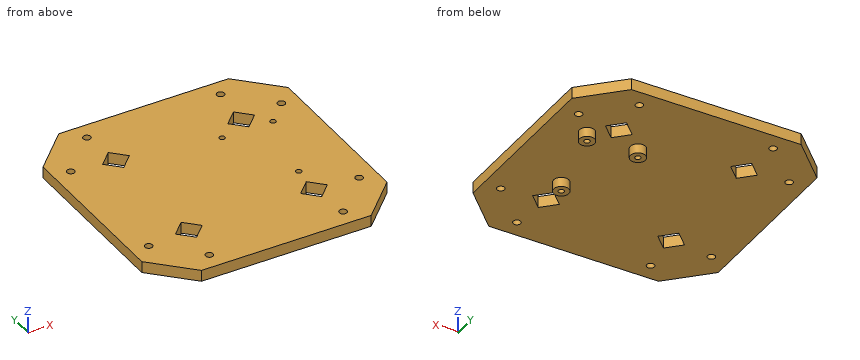
```python
from build123d import *

# Parameters (mm, degrees)
SKETCH_1_W          = 130
SKETCH_1_H          = 130
EXTRUDE_1_DEPTH     = 6
CUT_EXTRUDE_1_DEPTH = 6
CUT_EXTRUDE_2_REACH = 185.946
SKETCH_11_R         = 2
CHAMFER_1_SIZE      = 20
CUT_EXTRUDE_3_REACH = 185.946
SKETCH_12_R         = 1.5
SKETCH_13_R         = 4
SKETCH_13_R_2       = 1.5
EXTRUDE_2_DEPTH     = 5


with BuildPart() as part:
    # 草圖1 → 填料-伸長1 (new body)
    with BuildSketch(Plane.XY):
        with Locations((-65, 65)):
            Rectangle(SKETCH_1_W, SKETCH_1_H)
    extrude(amount=EXTRUDE_1_DEPTH)

    # 草圖10 → 除料-伸長1 (cut)
    with BuildSketch(Plane.XY.offset(6)):
        Polygon((-38.890872965, 98.180194847), (-31.819805153, 105.251262658), (-24.748737342, 98.180194847), (-31.819805153, 91.109127035), align=None)
        Polygon((-98.180194847, 105.251262658), (-105.251262658, 98.180194847), (-98.180194847, 91.109127035), (-91.109127035, 98.180194847), align=None)
        Polygon((-91.109127035, 31.819805153), (-98.180194847, 24.748737342), (-105.251262658, 31.819805153), (-98.180194847, 38.890872965), align=None)
        Polygon((-31.819805153, 24.748737342), (-24.748737342, 31.819805153), (-31.819805153, 38.890872965), (-38.890872965, 31.819805153), align=None)
    extrude(amount=-CUT_EXTRUDE_1_DEPTH, mode=Mode.SUBTRACT)

    # 草圖11 → 除料-伸長2 (cut, up to next)
    with BuildSketch(Plane.XY.offset(6), mode=Mode.PRIVATE) as cut_extrude_2_sk1:
        with Locations((-9.2, 100.435324702)):
            Circle(SKETCH_11_R)
    cut_extrude_2_tool1 = extrude(cut_extrude_2_sk1.sketch, amount=-CUT_EXTRUDE_2_REACH, mode=Mode.PRIVATE) & part.part
    # 草圖11 → 除料-伸長2 (cut, up to next)
    with BuildSketch(Plane.XY.offset(6), mode=Mode.PRIVATE) as cut_extrude_2_sk2:
        with Locations((-29.564675298, 120.8)):
            Circle(SKETCH_11_R)
    cut_extrude_2_tool2 = extrude(cut_extrude_2_sk2.sketch, amount=-CUT_EXTRUDE_2_REACH, mode=Mode.PRIVATE) & part.part
    # 草圖11 → 除料-伸長2 (cut, up to next)
    with BuildSketch(Plane.XY.offset(6), mode=Mode.PRIVATE) as cut_extrude_2_sk3:
        with Locations((-100.435324702, 120.8)):
            Circle(SKETCH_11_R)
    cut_extrude_2_tool3 = extrude(cut_extrude_2_sk3.sketch, amount=-CUT_EXTRUDE_2_REACH, mode=Mode.PRIVATE) & part.part
    # 草圖11 → 除料-伸長2 (cut, up to next)
    with BuildSketch(Plane.XY.offset(6), mode=Mode.PRIVATE) as cut_extrude_2_sk4:
        with Locations((-120.8, 100.435324702)):
            Circle(SKETCH_11_R)
    cut_extrude_2_tool4 = extrude(cut_extrude_2_sk4.sketch, amount=-CUT_EXTRUDE_2_REACH, mode=Mode.PRIVATE) & part.part
    # 草圖11 → 除料-伸長2 (cut, up to next)
    with BuildSketch(Plane.XY.offset(6), mode=Mode.PRIVATE) as cut_extrude_2_sk5:
        with Locations((-120.8, 29.564675298)):
            Circle(SKETCH_11_R)
    cut_extrude_2_tool5 = extrude(cut_extrude_2_sk5.sketch, amount=-CUT_EXTRUDE_2_REACH, mode=Mode.PRIVATE) & part.part
    # 草圖11 → 除料-伸長2 (cut, up to next)
    with BuildSketch(Plane.XY.offset(6), mode=Mode.PRIVATE) as cut_extrude_2_sk6:
        with Locations((-100.435324702, 9.2)):
            Circle(SKETCH_11_R)
    cut_extrude_2_tool6 = extrude(cut_extrude_2_sk6.sketch, amount=-CUT_EXTRUDE_2_REACH, mode=Mode.PRIVATE) & part.part
    # 草圖11 → 除料-伸長2 (cut, up to next)
    with BuildSketch(Plane.XY.offset(6), mode=Mode.PRIVATE) as cut_extrude_2_sk7:
        with Locations((-29.564675298, 9.2)):
            Circle(SKETCH_11_R)
    cut_extrude_2_tool7 = extrude(cut_extrude_2_sk7.sketch, amount=-CUT_EXTRUDE_2_REACH, mode=Mode.PRIVATE) & part.part
    # 草圖11 → 除料-伸長2 (cut, up to next)
    with BuildSketch(Plane.XY.offset(6), mode=Mode.PRIVATE) as cut_extrude_2_sk8:
        with Locations((-9.2, 29.564675298)):
            Circle(SKETCH_11_R)
    cut_extrude_2_tool8 = extrude(cut_extrude_2_sk8.sketch, amount=-CUT_EXTRUDE_2_REACH, mode=Mode.PRIVATE) & part.part
    add(cut_extrude_2_tool1.solids().sort_by_distance((-9.2, 100.435325, 6))[0], mode=Mode.SUBTRACT)
    add(cut_extrude_2_tool2.solids().sort_by_distance((-29.564675, 120.8, 6))[0], mode=Mode.SUBTRACT)
    add(cut_extrude_2_tool3.solids().sort_by_distance((-100.435325, 120.8, 6))[0], mode=Mode.SUBTRACT)
    add(cut_extrude_2_tool4.solids().sort_by_distance((-120.8, 100.435325, 6))[0], mode=Mode.SUBTRACT)
    add(cut_extrude_2_tool5.solids().sort_by_distance((-120.8, 29.564675, 6))[0], mode=Mode.SUBTRACT)
    add(cut_extrude_2_tool6.solids().sort_by_distance((-100.435325, 9.2, 6))[0], mode=Mode.SUBTRACT)
    add(cut_extrude_2_tool7.solids().sort_by_distance((-29.564675, 9.2, 6))[0], mode=Mode.SUBTRACT)
    add(cut_extrude_2_tool8.solids().sort_by_distance((-9.2, 29.564675, 6))[0], mode=Mode.SUBTRACT)

    # 導角1
    chamfer_1_edges = [part.edges().sort_by_distance(p)[0] for p in [
        (-130, 0, 3),
        (-130, 130, 3),
        (0, 130, 3),
        (0, 0, 3),
    ]]
    chamfer(chamfer_1_edges, length=CHAMFER_1_SIZE)

    # 草圖12 → 除料-伸長3 (cut, up to next)
    with BuildSketch(Plane.XY.offset(6), mode=Mode.PRIVATE) as cut_extrude_3_sk1:
        with Locations((-47, 89.5)):
            Circle(SKETCH_12_R)
    cut_extrude_3_tool1 = extrude(cut_extrude_3_sk1.sketch, amount=-CUT_EXTRUDE_3_REACH, mode=Mode.PRIVATE) & part.part
    # 草圖12 → 除料-伸長3 (cut, up to next)
    with BuildSketch(Plane.XY.offset(6), mode=Mode.PRIVATE) as cut_extrude_3_sk2:
        with Locations((-20, 89.5)):
            Circle(SKETCH_12_R)
    cut_extrude_3_tool2 = extrude(cut_extrude_3_sk2.sketch, amount=-CUT_EXTRUDE_3_REACH, mode=Mode.PRIVATE) & part.part
    # 草圖12 → 除料-伸長3 (cut, up to next)
    with BuildSketch(Plane.XY.offset(6), mode=Mode.PRIVATE) as cut_extrude_3_sk3:
        with Locations((-30.5, 48)):
            Circle(SKETCH_12_R)
    cut_extrude_3_tool3 = extrude(cut_extrude_3_sk3.sketch, amount=-CUT_EXTRUDE_3_REACH, mode=Mode.PRIVATE) & part.part
    add(cut_extrude_3_tool1.solids().sort_by_distance((-47, 89.5, 6))[0], mode=Mode.SUBTRACT)
    add(cut_extrude_3_tool2.solids().sort_by_distance((-20, 89.5, 6))[0], mode=Mode.SUBTRACT)
    add(cut_extrude_3_tool3.solids().sort_by_distance((-30.5, 48, 6))[0], mode=Mode.SUBTRACT)

    # 草圖13 → 填料-伸長2 (add)
    # profile 1 of 3: a face of its own
    with BuildSketch(Plane(origin=(0, 0, 0), x_dir=(-1, 0, 0), z_dir=(0, 0, -1))):
        with Locations(Location((20, 89.5, 0), (0, 0, 180))):
            Circle(SKETCH_13_R)
        with Locations(Location((20, 89.5, 0), (0, 0, 180))):
            Circle(SKETCH_13_R_2, mode=Mode.SUBTRACT)
    # profile 2 of 3: a face of its own
    with BuildSketch(Plane(origin=(0, 0, 0), x_dir=(-1, 0, 0), z_dir=(0, 0, -1))):
        with Locations(Location((47, 89.5, 0), (0, 0, 180))):
            Circle(SKETCH_13_R)
        with Locations(Location((47, 89.5, 0), (0, 0, 180))):
            Circle(SKETCH_13_R_2, mode=Mode.SUBTRACT)
    # profile 3 of 3: a face of its own
    with BuildSketch(Plane(origin=(0, 0, 0), x_dir=(-1, 0, 0), z_dir=(0, 0, -1))):
        with Locations(Location((30.5, 48, 0), (0, 0, 180))):
            Circle(SKETCH_13_R)
        with Locations(Location((30.5, 48, 0), (0, 0, 180))):
            Circle(SKETCH_13_R_2, mode=Mode.SUBTRACT)
    extrude(amount=EXTRUDE_2_DEPTH)


solid = part.part
```
The model under review builds one solid part; all positions refer to its coordinate system, in mm. Round coordinates to 2 decimals unless told otherwise and drop trailing zeros. Write each loop counter-clockwise with the first axis right and the second up, starting at its lowest first coordinate (ties: lowest second). Pieces come first, ordered by that corner, then holes. Notation, with made-up numbers: M 9,74 L 29,74 A28 cw 29,111 Z; hole C 58,-14.75 d1. An arc over 180 degrees is marked long. Use CSV: the item, a comma, the result in double quotes. Start each with the question number.
(1) We need section D-D, the plane x = -47. State the section outline as (y, z) points, then the cut area to 3 significant figures.
(2) Clearance check with flat-ended pins moving along their axes: P1, Ø4.5, axis at x = -29.56, y = 9.2, coming from the +Z side; P2, Ø5, axis at x = -17, z = 2, coming from the -Y side; P3, Ø5, axis at x = -29.56, y = 120.8, coming from the -Z side. State where each tip first meets the part, or that it passes through.
(3) We need section B-B, the plane y = 89.5. State the section outline as (x, z) points.
(4) We need section A-A, the plane x = -9.2. State the section outline as (y, z) points, then the cut area to 3 significant figures.
(5) We need section C-C, the plane z = -3. State the section outline as (x, y) points.
(6) For line 1 along X through (y, z) = (48, -2.65); line 2 along X through (y, z) = (120.5, 4.25); line 3 along Y through (x, z) = (-35.5, 1.25), list the stretches that pass through material, from the lowest coordinate up.
Findings:
1,outline,"M 0,0 L 85.5,0 L 85.5,-5 L 88,-5 L 88,6 L 0,6 Z; M 91,-5 L 93.5,-5 L 93.5,0 L 130,0 L 130,6 L 91,6 Z"
1,area,"787 mm^2"
2,P1,"z = 6"
2,P2,"y = 0.5"
2,P3,"z = 0"
3,outline,"M -130,0 L -51,0 L -51,-5 L -48.5,-5 L -48.5,6 L -130,6 Z; M -45.5,-5 L -43,-5 L -43,0 L -24,0 L -24,-5 L -21.5,-5 L -21.5,6 L -45.5,6 Z; M -18.5,-5 L -16,-5 L -16,0 L 0,0 L 0,6 L -18.5,6 Z"
4,outline,"M 10.8,0 L 27.56,0 L 27.56,6 L 10.8,6 Z; M 31.56,0 L 98.44,0 L 98.44,6 L 31.56,6 Z; M 102.44,0 L 119.2,0 L 119.2,6 L 102.44,6 Z"
4,area,"602 mm^2"
5,outline,"C -47,89.5 d8; C -30.5,48 d8; C -20,89.5 d8; hole C -47,89.5 d3; hole C -30.5,48 d3; hole C -20,89.5 d3"
6,line 1,"-34.5 to -32, -29 to -26.5"
6,line 2,"-119.5 to -102.41, -98.46 to -31.54, -27.59 to -10.5"
6,line 3,"0 to 28.43, 35.21 to 94.79, 101.57 to 130"
